Print and shaded views of the part. All mm, measured from the part's lowest x, y and z. Round coordinates to 2 decimals unless told otherwise and drop trailing zeros. Loops run counter-clockwise (first coordinate to the right, second up) from the corner with the lowest first, then second, coordinate; pieces in that order, holes last. Notation, with made-up numbers: (77, -19) -> (113, -19) arc R18 ccw to (113, 2) -> close; hole circle Ø11 at (-3.5, 67.25). An arc over 180 degrees is marked (long way). Answer as CSV lines item,"result".
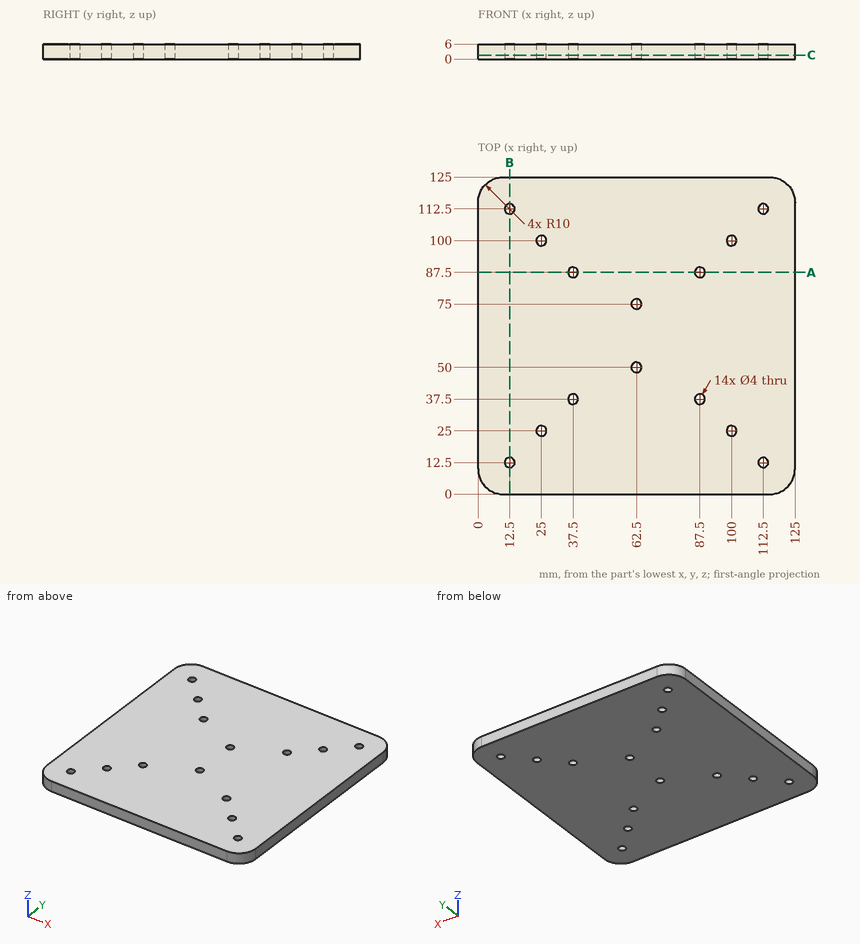
Q1. Drop flat-ended pins along their axis: P1, Ø3, axis at x = 12.5, y = 112.5, coming from the +Z side; P2, Ø4.5, axis at x = 112.5, y = 12.5, coming from the +Z side. Give the stop position or say it passes through.
Geometry results:
P1,"through"
P2,"z = 6"
Q2. Saw through at B-B, the plane x = 12.5. Write the cut outline in (y, z), then the cut area to 3 significant figures.
Geometry results:
outline,"(0, 0) -> (10.5, 0) -> (10.5, 6) -> (0, 6) -> close; (14.5, 0) -> (110.5, 0) -> (110.5, 6) -> (14.5, 6) -> close; (114.5, 0) -> (125, 0) -> (125, 6) -> (114.5, 6) -> close"
area,"702 mm2"
Q3. Saw through at C-C, the plane z = 1.65. Give the number of separate pieces and of enclosed holes in the cut face, then the cut area to 3 significant figures.
Geometry results:
separate pieces,"1"
enclosed holes,"14"
area,"15,400 mm2"
Q4. Drill centre lines: line 1 along Y through (x, z) = (87.5, 1.75); line 2 along X through (y, z) = (100, 1.45). Where is each one in solid material? Low to high.
Geometry results:
line 1,"0 to 35.5, 39.5 to 85.5, 89.5 to 125"
line 2,"0 to 23, 27 to 98, 102 to 125"
Q5. Saw through at A-A, the plane y = 87.5. Write the cut outline in (x, z), then the cut area to 3 significant figures.
Geometry results:
outline,"(0, 0) -> (35.5, 0) -> (35.5, 6) -> (0, 6) -> close; (39.5, 0) -> (85.5, 0) -> (85.5, 6) -> (39.5, 6) -> close; (89.5, 0) -> (125, 0) -> (125, 6) -> (89.5, 6) -> close"
area,"702 mm2"
